from build123d import *

# Parameters (mm, degrees)
BOSS_EXTRUDE1_DEPTH = 2.75
SKETCH3_R           = 1.7
CUT_EXTRUDE1_DEPTH  = 2.75
BOSS_EXTRUDE2_DEPTH = 4.45
SKETCH6_R           = 5.435
BOSS_EXTRUDE3_DEPTH = 3.3


with BuildPart() as part:
    # Sketch2 → Boss-Extrude1 (new body)
    with BuildSketch(Plane.XY):
        with BuildLine():
            add(Edge.make_bspline(
                [(4.61101002, 8.44423368), (6.970103918, 8.506940606), (9.06101002, 7.719664696)],
                knots=[0, 0, 0, 0.687711527, 0.687711527, 0.687711527], degree=2))
            Line((9.06101002, 7.719664696), (9.06101002, 7.219432127))
            Line((9.06101002, 7.219432127), (21.36101002, 6.84423368))
            ThreePointArc((21.36101002, 6.84423368), (25.56101002, 2.64423368), (21.36101002, -1.55576632))
            Line((21.36101002, -1.55576632), (9.06101002, -1.930964768))
            Line((9.06101002, -1.930964768), (9.06101002, -2.431197337))
            add(Edge.make_bspline(
                [(4.61101002, -3.15576632), (6.970103918, -3.218473247), (9.06101002, -2.431197337)],
                knots=[0, 0, 0, 0.687711527, 0.687711527, 0.687711527], degree=2))
            add(Edge.make_bspline(
                [(4.61101002, -3.15576632), (2.251916122, -3.218473247), (0.16101002, -2.431197337)],
                knots=[0, 0, 0, 0.687711527, 0.687711527, 0.687711527], degree=2))
            Line((0.16101002, -2.431197337), (0.16101002, -1.930964768))
            Line((0.16101002, -1.930964768), (-12.13898998, -1.55576632))
            ThreePointArc((-12.13898998, -1.55576632), (-16.33898998, 2.64423368), (-12.13898998, 6.84423368))
            Line((-12.13898998, 6.84423368), (0.16101002, 7.219432127))
            Line((0.16101002, 7.219432127), (0.16101002, 7.719664696))
            add(Edge.make_bspline(
                [(4.61101002, 8.44423368), (2.251916122, 8.506940606), (0.16101002, 7.719664696)],
                knots=[0, 0, 0, 0.687711527, 0.687711527, 0.687711527], degree=2))
        make_face()
    extrude(amount=BOSS_EXTRUDE1_DEPTH)

    # Sketch3 → Cut-Extrude1 (cut)
    with BuildSketch(Plane.XY.offset(2.75)):
        with Locations((-11.88898998, 2.645532794)):
            Circle(SKETCH3_R)
        with Locations(Location((21.11101002, 2.645532794, 0), (0, 0, 180))):
            Circle(SKETCH3_R)
    extrude(amount=-CUT_EXTRUDE1_DEPTH, mode=Mode.SUBTRACT)

    # Sketch5 → Boss-Extrude2 (add)
    with BuildSketch(Plane.XY.offset(2.75)):
        with BuildLine():
            Line((9.06101002, 7.719664696), (9.06101002, 7.219432127))
            Line((9.06101002, 7.219432127), (9.06101002, -1.930964768))
            Line((9.06101002, -1.930964768), (9.06101002, -2.431197337))
            add(Edge.make_bspline(
                [(4.61101002, -3.15576632), (6.970103918, -3.218473247), (9.06101002, -2.431197337)],
                knots=[0, 0, 0, 1, 1, 1], degree=2))
            add(Edge.make_bspline(
                [(4.61101002, -3.15576632), (2.251916122, -3.218473247), (0.16101002, -2.431197337)],
                knots=[0, 0, 0, 1, 1, 1], degree=2))
            Line((0.16101002, -2.431197337), (0.16101002, -1.930964768))
            Line((0.16101002, -1.930964768), (0.16101002, 7.219432127))
            Line((0.16101002, 7.219432127), (0.16101002, 7.719664696))
            add(Edge.make_bspline(
                [(4.61101002, 8.44423368), (2.251916122, 8.506940606), (0.16101002, 7.719664696)],
                knots=[0, 0, 0, 1, 1, 1], degree=2))
            add(Edge.make_bspline(
                [(4.61101002, 8.44423368), (6.970103918, 8.506940606), (9.06101002, 7.719664696)],
                knots=[0, 0, 0, 1, 1, 1], degree=2))
        make_face()
    extrude(amount=BOSS_EXTRUDE2_DEPTH)

    # Sketch6 → Boss-Extrude3 (add)
    with BuildSketch(Plane.XY.offset(7.2)):
        with Locations(Location((4.611010009, 2.647143575, 0), (0, 0, 215.038419813))):
            Circle(SKETCH6_R)
    extrude(amount=BOSS_EXTRUDE3_DEPTH)


solid = part.part
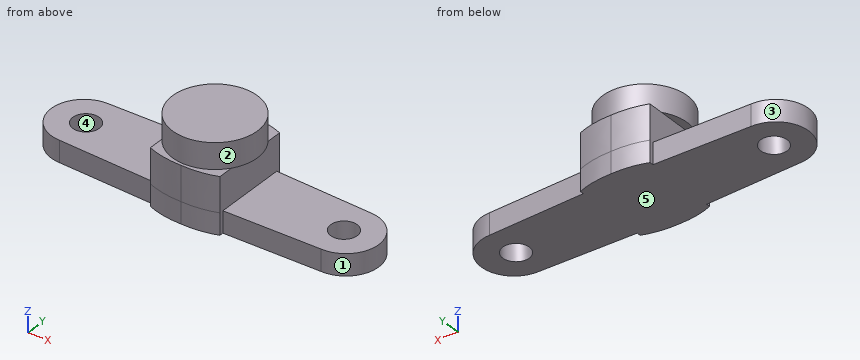
The listing builds one solid part. Answer for the finished solid, in the listing's coordinates (mm). Face numbers are marked on the shaded views. A direction names the side the tool comes from. Coordinates: 2 decimals unless noted, no trailing zeros. Write each loop counter-clockwise with the first axis right and the second up, starting at its lowest first coordinate (ties: lowest second). Pieces come first, ordered by that corner, then holes. Notation, with made-up numbers: M 65,84.25 L 89,84.25 A4 ccw 89,88.25 Z; hole C 40,65 d9. An arc over 180 degrees is marked long. Put each result on its own line as item: value. Start each with the question number.
1. A cutting plane is placed at C-C on z = 8.25. Write down the section's boundary in (x, y) (3 decimals).
2. A cutting plane is placed at B-B on y = 2.25. Write down the section's boundary in (x, z), then the cut area to 3 significant figures.
3. Consider line 1 (X direction, y = 5, z = 7); line 2 (Z direction, x = 20.5, y = -1); line 3 (Y direction, x = 6, z = 8.75). Determine where each line is inside the solid, lowest interval first. Write a range as from..to.
4. Flat-ended cylindrical pins translate along their axes: P1, Ø1, axis at x = 11.5, z = 2, coming from the +Y side; P2, Ø6, axis at x = -2, z = 6, coming from the -Y side; P3, Ø2, axis at y = 1, z = 2, coming from the +X side; P4, Ø2.5, axis at x = -11.89, y = 2.65, coming from the +Z side. Find the tip coordinate at first contact, or state that the pin passes through.
5. For a pull along Y with two mould halves and no side action, classify the marked faces 3, 4 and 5 as pulls with the +Y half, pulls with the -Y half, needs draft (parallel to the pull), parting line crosses it, or undercut.
6. A cutting plane is placed at A-A on x = 20. Write down the section's boundary in (y, z).
7. A cutting plane is placed at D-D on y = 5.25. Write down the section's boundary in (x, z), then the cut area to 3 significant figures.
8. Which of the six approach directions +Z, -Z, +X, -X, +Y, -Y give full straight-line access (tool end or side, diameter ignored) to the marked faces 1 and 2?
Resolved:
1. outline: C 4.611,2.647 d10.87
2. outline: M -16.32,0 L -13.54,0 L -13.54,2.75 L -16.32,2.75 Z; M -10.24,0 L 19.46,0 L 19.46,2.75 L 9.06,2.75 L 9.06,7.2 L 10.03,7.2 L 10.03,10.5 L -0.81,10.5 L -0.81,7.2 L 0.16,7.2 L 0.16,2.75 L -10.24,2.75 Z; M 22.76,0 L 25.54,0 L 25.54,2.75 L 22.76,2.75 Z
2. area: 172 mm2
3. line 1: x = 0.16..9.06
3. line 2: z = 0..2.75
3. line 3: y = -2.61..7.9
4. P1: stops at y = 7.16
4. P2: stops at y = -2.71
4. P3: stops at x = 25.51
4. P4: passes through
5. face 3: parting line crosses it
5. face 4: undercut
5. face 5: needs draft
6. outline: M -1.6,0 L 1.36,0 L 1.36,2.75 L -1.6,2.75 Z; M 3.93,0 L 6.89,0 L 6.89,2.75 L 3.93,2.75 Z
7. outline: M -15.43,0 L 24.65,0 L 24.65,2.75 L 9.06,2.75 L 9.06,7.2 L 9.38,7.2 L 9.38,10.5 L -0.16,10.5 L -0.16,7.2 L 0.16,7.2 L 0.16,2.75 L -15.43,2.75 Z
7. area: 181 mm2
8. face 1: +Z, -Z, +X
8. face 2: +Z
